Design review of the part built by this model. Coordinates are the model's own, in mm. A direction names the side the tool comes from. Coordinates: 2 decimals unless noted, no trailing zeros. Loops run counter-clockwise (first coordinate to the right, second up) from the corner with the lowest first, then second, coordinate; pieces in that order, holes last. Notation, with made-up numbers: (57, 1.25) -> (116, 1.25) arc R27 cw to (116, 39.25) -> close; hole circle Ø1 at (70.25, -19.5). An arc over 180 degrees is marked (long way). One line per item, written item: value. Start each with the question number.
1. Add section C-C on z = -10.25. Write out the cut boundary in (x, y), plus the area to 3 significant figures.
2. Add section B-B on y = 0. Write out the cut boundary in (x, z), plus the area to 3 significant figures.
3. Insertion check: pin 1 (4 mm diameter, centred on x = -2, z = -18, fed in from +Y); pin 2 (5 mm diameter, centred on y = 3, z = -6, fed in from -X); pin 3 (0.5 mm diameter, centred on x = 0.5, z = -0.5, fed in from +Y). Each pin has a flat end and moves straight along its axis. Give the tip position at first contact, or say it passes through.
4. For probe 1 along Y at (x, z) = (1.5, -10); probe 2 along X at (y, z) = (-1, -7), list the stretches that pass through material, from the lowest coordinate up.
5. Add section A-A on x = 0. Write out the cut boundary in (y, z), plus the area to 3 significant figures.
6. Machinability: for faces 1 (the flat face through (-0.1, -0.4, -0.5)), 2 (the cylindrical face through (-2.685, -0.596, -11.372)), 3 (the flat face through (0, 2, 0)), which of the approach directions +Z, -Z, +X, -X, +Y, -Y give a long, thin tool a straight path to every point of the face, cutting with its end or side? Answer none if there is none.
Solid Edge part; units mm, degrees
sketch "Sketch1" plane through (0, 0, 0) normal (0, 0, 1) x (1, 0, 0)
  circle A0 centre (0, 0) radius 4.75
extrude "拉伸_4" add sketch "Sketch1" against normal blind 2.7
sketch "Sketch2" plane through (0, 0, 0) normal (0, 0, 1) x (1, 0, 0)
  line L0 (-5, -0.4) -> (5, -0.4)
  line L1 (5, -0.4) -> (5, 0.4)
  line L2 (5, 0.4) -> (-5, 0.4)
  line L3 (-5, 0.4) -> (-5, -0.4)
extrude "拉伸除料_2" cut sketch "Sketch2" against normal blind 1
sketch "Sketch3" plane through (0, 0, 0) normal (1, 0, 0) x (0, 1, 0)
  line L0 (4.75, -0.5) -> (2.55, -2.7)
  line L1 (2.55, -2.7) -> (5.5063, -2.7)
  line L2 (5.5063, -2.7) -> (4.75, -0.5)
revolve "RevolvedCutout1" cut sketch "Sketch3" angle 360 about axis through (0, 0, 0) along (0, 0, -1)
sketch "Sketch4" plane through (0, 0, -2.7) normal (0, 0, -1) x (0, 1, 0)
  circle A0 centre (0, 0) radius 2.75
extrude "拉伸_6" add sketch "Sketch4" along normal blind 17.3 and the other way blind 0.4309
cosmetic_thread "Thread1"
properties material "不锈钢310"
Worked answers:
1. outline: circle Ø5.5 at (0, 0)
1. area: 23.8 mm²
2. outline: (-4.25, -1) -> (-2.75, -2.5) -> (-2.75, -20) -> (2.75, -20) -> (2.75, -2.5) -> (4.25, -1) -> close
2. area: 107 mm²
3. pin 1: stops at y = 2.75
3. pin 2: stops at x = -2.7
3. pin 3: stops at y = 4.74
4. probe 1: y = -2.3 to 2.3
4. probe 2: x = -2.56 to 2.56
5. outline: (-4.75, -0.5) -> (-2.75, -2.5) -> (-2.75, -20) -> (2.75, -20) -> (2.75, -2.5) -> (4.75, -0.5) -> (4.75, 0) -> (0.4, 0) -> (0.4, -1) -> (-0.4, -1) -> (-0.4, 0) -> (-4.75, 0) -> close
5. area: 115 mm²
6. face 1: +Z, +X, -X
6. face 2: -Z
6. face 3: +Z, +X, -X, +Y, -Y
